Part model, mm, in its own coordinate system. Face numbers are marked on the shaded views. A direction names the side the tool comes from. Give positions to 0.01 mm unless a question says otherwise; leave off trailing zeros. Order: outer loops, then holes, each group sorted by start corner. A loop starts at its lowest first (then second) coordinate and runs counter-clockwise, first axis right, second up. Notation, with made-up numbers: (85.5, -3.5) -> (114.5, -3.5) arc R28 cw to (114.5, 26.5) -> close; hole circle Ø10 at (-29, 35). An arc over 180 degrees is marked (long way). Write item = value, one per line. Start each with the question number.
Item 1: Flat gauge pins, fed straight in: P1, Ø6, axis at x = -10.5, y = 15.5, coming from the +Z side; P2, Ø5.5, axis at y = 22.5, z = -7.5, coming from the +X side; P3, Ø8, axis at x = -9, z = 3, coming from the +Y side; P4, Ø12, axis at x = 12.5, y = 20.5, coming from the -Z side. Where does each tip first touch, or does it go through?
Item 2: Band-saw the part on A-A on x = 0. Write the cut outline in (y, z), plus the area to 3 significant figures.
Item 3: Pull direction Y, two halves, no side cores. Call the marked faces 1, 2 and 3: +Y half, -Y half, draft (parallel to the pull), parting line (faces both ways), or undercut.
Item 4: Band-saw the part on B-B on z = 0. Write the cut outline in (x, y), plus the area to 3 significant figures.
Item 5: Drill centre lines: line 1 along Y through (x, z) = (15, -6.45); line 2 along Z through (x, y) = (0, 4); line 3 along Y through (x, z) = (8, -5.25). Where is each one in solid material? Low to high.
Item 6: Tool access for the marked faces 4, 5 and 6: list every direction of +Z, -Z, +X, -X, +Y, -Y with a clear straight run to the whole face (end or side of a thin tool).
Item 7: Band-saw the part on C-C on y = 4. Write the cut outline in (x, z).
Item 8: Band-saw the part on D-D on x = 15. Write the cut outline in (y, z), plus the area to 3 significant figures.
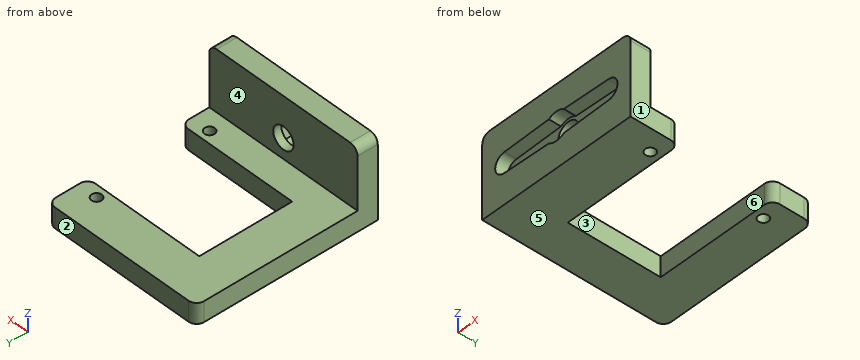
Autodesk Inventor part; units mm, degrees
ref_plane "YZ Plane" through (0, 0, 0) normal (1, 0, 0) x (0, 1, 0)
ref_plane "XZ Plane" through (0, 0, 0) normal (0, 1, 0) x (-1, 0, 0)
ref_plane "XY Plane" through (0, 0, 0) normal (0, 0, 1) x (1, 0, 0)
sketch "Sketch1" plane through (0, 0, 0) normal (0, 1, 0) x (-1, 0, 0)
  line L0 (-20, 20) -> (20, 20)
  line L1 (20, 20) -> (20, -20)
  line L2 (20, -20) -> (-20, -20)
  line L3 (-20, -20) -> (-20, 20)
  line L4 (-20, 20) -> (20, -20) construction
  line L5 (20, 20) -> (-20, -20) construction
  point P0 (0, 0)
  dimension "d0" = 40
  dimension "d1" = 40
extrude "Extrusion1" add sketch "Sketch1" along normal blind 5
sketch "Sketch4" plane through (0, 5, 0) normal (0, 1, 0) x (1, 0, 0)
  line L0 (-20, 10) -> (-10, 10)
  line L1 (-10, 10) -> (-10, 5)
  line L2 (-10, 5) -> (-20, 5)
  line L3 (-20, 5) -> (-20, 10)
  line L4 (-20, 10) -> (-10, 5) construction
  line L5 (-10, 10) -> (-20, 5) construction
  line L6 (-20, -20) -> (20, -20)
  line L7 (20, -20) -> (20, 20)
  line L8 (-20, 20) -> (-20, -20)
  point P0 (-15, 7.5)
  dimension "d20" = 10
  dimension "d21" = 5
  dimension "d23" = 25
extrude "Extrusion4" add sketch "Sketch4" along normal blind 40
sketch "Sketch8" plane through (-10, 5, -5) normal (1, 0, 0) x (0, 0, -1)
  line L0 (0, 40) -> (5, 40)
  line L1 (5, 40) -> (5, 30)
  line L2 (5, 30) -> (0, 30)
  line L3 (0, 30) -> (0, 40)
  line L4 (0, 7) -> (5, 7)
  line L5 (5, 7) -> (5, 0)
  line L6 (5, 0) -> (0, 0)
  line L7 (0, 0) -> (0, 7)
  line L8 (5, 0) -> (5, 40)
  line L9 (0, 40) -> (5, 40)
  point P0 (-5, -5)
  dimension "d44" = 5
  dimension "d45" = 10
  dimension "d46" = 5
  dimension "d47" = 7
  dimension "d48" = 23
extrude "Extrusion7" add sketch "Sketch8" along normal blind 30
sketch "Sketch9" plane through (-20, 5, -5) normal (0, 0, 1) x (1, 0, 0)
  circle A0 centre (35, 32.5) radius 1.25
  circle A1 centre (35, 4.5) radius 1.25
  line L0 (10, 30) -> (40, 30)
  line L1 (40, 40) -> (40, 30)
  line L2 (40, 7) -> (40, 0)
  point P0 (20, -5)
  dimension "d51" = 2.5
  dimension "d52" = 2.5
  dimension "d53" = 28
  dimension "d54" = 2.5
  dimension "d55" = 5
  dimension "d56" = 5
extrude "Extrusion8" cut sketch "Sketch9" against normal blind 5
sketch "Sketch11" plane through (0, 5, 0) normal (0, 1, 0) x (1, 0, 0)
  line L0 (20, -20) -> (-20, -20)
  line L1 (-20, -20) -> (-20, -10)
  line L2 (-20, -10) -> (20, -10)
  line L3 (20, -10) -> (20, -20)
  line L4 (-20, 10) -> (20, 10)
  line L5 (20, 10) -> (20, 20)
  line L6 (20, 20) -> (-20, 20)
  line L7 (-20, 20) -> (-20, 10)
  line L8 (20, 20) -> (-20, 20)
  line L9 (-20, -20) -> (20, -20)
  line L10 (20, -20) -> (20, 5)
  line L11 (20, 10) -> (20, 20)
  point P0 (0, 0)
  dimension "d59" = 40
  dimension "d60" = 10
  dimension "d61" = 40
  dimension "d62" = 10
extrude "Extrusion9" cut sketch "Sketch11" against normal blind 5
sketch "Sketch12" plane through (0, 0, 0) normal (0, -1, 0) x (1, 0, 0)
  circle A0 centre (0, 0) radius 3.5
  circle A1 centre (14, 0) radius 2.5
  circle A2 centre (-14, 0) radius 2.5
  line L0 (-20, -10) -> (20, -10)
  line L1 (-14, 2.5) -> (-2.0057, 2.8683)
  line L2 (-14, -2.5) -> (-2.0057, -2.8683)
  line L3 (14, 2.5) -> (2.0057, 2.8683)
  line L4 (14, -2.5) -> (2.0057, -2.8683)
  dimension "d65" = 7
  dimension "d66" = 5
  dimension "d67" = 5
  dimension "d68" = 14
  dimension "d69" = 10
  dimension "d70" = 10
  dimension "d71" = 14
  dimension "d72" = 12
  dimension "d73" = 12
extrude "Extrusion10" cut sketch "Sketch12" against normal blind 3
sketch "Sketch13" plane through (0, 3, 0) normal (0, -1, 0) x (1, 0, 0)
  circle A0 centre (0, 0) radius 2.75
  dimension "d76" = 5.5
extrude "Extrusion11" cut sketch "Sketch13" against normal blind 3
fillet "Fillet1" radius 2 6 edges at (20, 45, -7.5) (20, 35, -7.5) (20, 12, -7.5) (20, 2.5, 10) (-20, 2.5, 10) (-20, 45, -7.5)
properties part number "head_bottom"
Values found:
q1.P1 = -5
q1.P2 = -10
q1.P3 = 5
q1.P4 = through
q2.outline = (0, -10) -> (12, -10) -> (12, -5) -> (5, -5) -> (5, -2.75) -> (3, -2.75) -> (3, -3.5) -> (0, -3.5) -> close; (0, 3.5) -> (3, 3.5) -> (3, 2.75) -> (5, 2.75) -> (5, 10) -> (0, 10) -> close; (35, -10) -> (45, -10) -> (45, -5) -> (35, -5) -> close
q2.area = 153 mm^2
q3.face_1 = draft
q3.face_2 = +Y half
q3.face_3 = undercut
q4.outline = (-20, 0) -> (-16.5, 0) -> (-16.5, 3) -> (-2.75, 3) -> (-2.75, 5) -> (-20, 5) -> close; (2.75, 3) -> (16.5, 3) -> (16.5, 0) -> (20, 0) -> (20, 5) -> (2.75, 5) -> close
q4.area = 90.0 mm^2
q5.line_1 = 0 to 8.25, 10.75 to 12, 35 to 36.25, 38.75 to 45
q5.line_2 = -10 to -2.75, 2.75 to 10
q5.line_3 = 0 to 12, 35 to 45
q6.face_4 = +Z, +X, -X, +Y
q6.face_5 = -Z, +X, -X, +Y, -Y
q6.face_6 = +Z, -Z, +X
q7.outline = (-20, -10) -> (20, -10) -> (20, 8) arc R2 ccw to (18, 10) -> (-18, 10) arc R2 ccw to (-20, 8) -> close; hole circle Ø5.5 at (0, 0)
q8.outline = (0, -10) -> (8.25, -10) -> (8.25, -5) -> (5, -5) -> (5, 10) -> (0, 10) -> (0, 2.29) -> (3, 2.29) -> (3, -2.29) -> (0, -2.29) -> close; (10.75, -10) -> (12, -10) -> (12, -5) -> (10.75, -5) -> close; (35, -10) -> (36.25, -10) -> (36.25, -5) -> (35, -5) -> close; (38.75, -10) -> (45, -10) -> (45, -5) -> (38.75, -5) -> close
q8.area = 146 mm^2
